```python
from build123d import *

# Parameters (mm, degrees)
BOSS_EXTRUDE1_DEPTH = 6.35
FILLET3_R           = 3.175


with BuildPart() as part:
    # Sketch2 → Boss-Extrude1 (new body)
    with BuildSketch(Plane.XY):
        with BuildLine():
            Line((0, 0), (0, 38.1))
            ThreePointArc((0, 38.1), (3.719743879, 47.080256121), (12.7, 50.8))
            Line((12.7, 50.8), (685.8, 50.8))
            ThreePointArc((685.8, 50.8), (694.780256121, 47.080256121), (698.5, 38.1))
            Line((698.5, 38.1), (698.5, 0))
            ThreePointArc((698.5, 0), (694.780256121, -8.980256121), (685.8, -12.7))
            Line((685.8, -12.7), (12.7, -12.7))
            ThreePointArc((12.7, -12.7), (3.719743879, -8.980256121), (0, 0))
        make_face()
        with BuildLine():
            Line((6.35, 38.1), (6.35, 0))
            ThreePointArc((6.35, 0), (8.209871939, -4.490128061), (12.7, -6.35))
            Line((12.7, -6.35), (685.8, -6.35))
            ThreePointArc((685.8, -6.35), (690.290128061, -4.490128061), (692.15, 0))
            Line((692.15, 0), (692.15, 38.1))
            ThreePointArc((692.15, 38.1), (690.290128061, 42.590128061), (685.8, 44.45))
            Line((685.8, 44.45), (12.7, 44.45))
            ThreePointArc((12.7, 44.45), (8.209871939, 42.590128061), (6.35, 38.1))
        make_face(mode=Mode.SUBTRACT)
    extrude(amount=BOSS_EXTRUDE1_DEPTH)

    # Fillet3
    fillet3_edges = [part.edges().sort_by_distance(p)[0] for p in [
        (0, 19.05, 6.35),
        (3.719743879, 47.080256121, 6.35),
        (349.25, 50.8, 6.35),
        (694.780256121, 47.080256121, 6.35),
        (698.5, 19.05, 6.35),
        (694.780256121, -8.980256121, 6.35),
        (349.25, -12.7, 6.35),
        (3.719743879, -8.980256121, 6.35),
        (0, 19.05, 0),
        (3.719743879, 47.080256121, 0),
        (349.25, 50.8, 0),
        (694.780256121, 47.080256121, 0),
        (698.5, 19.05, 0),
        (694.780256121, -8.980256121, 0),
        (349.25, -12.7, 0),
        (3.719743879, -8.980256121, 0),
        (349.25, 44.45, 6.35),
        (690.290128061, 42.590128061, 6.35),
        (692.15, 19.05, 6.35),
        (690.290128061, -4.490128061, 6.35),
        (349.25, -6.35, 6.35),
        (8.209871939, -4.490128061, 6.35),
        (6.35, 19.05, 6.35),
        (8.209871939, 42.590128061, 6.35),
        (349.25, 44.45, 0),
        (690.290128061, 42.590128061, 0),
        (692.15, 19.05, 0),
        (690.290128061, -4.490128061, 0),
        (349.25, -6.35, 0),
        (8.209871939, -4.490128061, 0),
        (6.35, 19.05, 0),
        (8.209871939, 42.590128061, 0),
    ]]
    fillet(fillet3_edges, radius=FILLET3_R - 0.0001)  # a hair under: the kernel refuses the full size


solid = part.part
```
Here's how the part is built. I have some questions about the finished solid (model axes, mm). Give positions to 0.01 mm unless a question says otherwise; leave off trailing zeros. Order: outer loops, then holes, each group sorted by start corner. A loop starts at its lowest first (then second) coordinate and runs counter-clockwise, first axis right, second up. Notation, with made-up numbers: M 62.5,46 L 91.5,46 A21 cw 91.5,54 Z; hole C 45.5,-39 d5. An arc over 180 degrees is marked long. Use a Markdown table: item, result. Add a question column.
1. I need wall thicknesses on probe 1 along Y at (x, z) = (596, 2.75); probe 2 along Y at (x, z) = (467, 4); probe 3 along X at (y, z) = (0.5, 2.75). Which ranges of each line are inside material? Lowest first, please. Write a range as from..to.
2. Suppose I cut it at C-C (z = 1.25). List the corners of the cut face in (x, y) for me, and give its area (3 significant figures).
3. For pin 1 Ø2 at (y, z) = (27, 2) entering from -X; pin 2 Ø1.5 at (x, z) = (420, 5) entering from +Y, each with a flat end and sliding along its axis, tell me the tip position at first contact or that it passes through.
Results list:
| question | item | result |
|---|---|---|
| 1 | probe 1 | y = -12.67..-6.38, 44.48..50.77 |
| 1 | probe 2 | y = -12.59..-6.46, 44.56..50.69 |
| 1 | probe 3 | x = 0.03..6.32, 692.18..698.47 |
| 2 | outline | M 0.65,0 A12.05 ccw 12.7,-12.05 L 685.8,-12.05 A12.05 ccw 697.85,0 L 697.85,38.1 A12.05 ccw 685.8,50.15 L 12.7,50.15 A12.05 ccw 0.65,38.1 Z; hole M 5.7,0 A7 ccw 12.7,-7 L 685.8,-7 A7 ccw 692.8,0 L 692.8,38.1 A7 ccw 685.8,45.1 L 12.7,45.1 A7 ccw 5.7,38.1 Z |
| 2 | area | 7,490 mm² |
| 3 | pin 1 | stops at x = 0 |
| 3 | pin 2 | stops at y = 50.61 |
